```python
from build123d import *

# Parameters (mm, degrees)
SKETCH_R  = 2.5
PAD_DEPTH = 0.8


with BuildPart() as part:
    # Sketch → Pad (new body)
    with BuildSketch(Plane.XY):
        with BuildLine():
            ThreePointArc((-3.20733, 0), (0, -3.20733), (3.20733, 0))
            Line((3.20733, 0), (3.20733, 29.5))
            Line((-3.20733, 29.5), (3.20733, 29.5))
            Line((-3.20733, 0), (-3.20733, 29.5))
        make_face()
        Circle(SKETCH_R, mode=Mode.SUBTRACT)
    extrude(amount=PAD_DEPTH)


solid = part.part
```
Source: CAD feature listing. Evaluate the final solid. Frame: model axes, mm. Give positions to 0.01 mm unless a question says otherwise; leave off trailing zeros. Write each loop counter-clockwise with the first axis right and the second up, starting at its lowest first coordinate (ties: lowest second). Pieces come first, ordered by that corner, then holes.
1. Section query B-B (z = 0.45). Return the cut outline in (x, y), then the cut area to 3 significant figures.
2. Section query A-A (x = 0). Return the cut outline in (y, z), then the cut area to 3 significant figures.
3. Material intervals for line 1 along Y through (x, z) = (0, 0.6); line 2 along Y through (x, z) = (1, 0.3); line 3 along X through (y, z) = (1, 0.7), sorted ascending.
4. Pull-direction query (Y, two-part tool) for faces 1 (the face through (0, 13, 0)), 2 (the face through (-0.54, -2.44, 0.39)), 3 (the face through (-0.071, -3.207, 0.394)); classes: +Y half, -Y half, draft (parallel to the pull), parting line (faces both ways), or undercut.
5. Section query C-C (x = -1.5). Return the cut outline in (y, z).
Output values:
1. outline: (-3.21, 0) arc R3.21 ccw to (3.21, 0) - (3.21, 29.5) - (-3.21, 29.5) - close; hole circle Ø5 at (0, 0)
1. area: 186 mm2
2. outline: (-3.21, 0) - (-2.5, 0) - (-2.5, 0.8) - (-3.21, 0.8) - close; (2.5, 0) - (29.5, 0) - (29.5, 0.8) - (2.5, 0.8) - close
2. area: 22.2 mm2
3. line 1: y = -3.21 to -2.5, 2.5 to 29.5
3. line 2: y = -3.05 to -2.29, 2.29 to 29.5
3. line 3: x = -3.21 to -2.29, 2.29 to 3.21
4. face 1: draft
4. face 2: undercut
4. face 3: -Y half
5. outline: (-2.83, 0) - (-2, 0) - (-2, 0.8) - (-2.83, 0.8) - close; (2, 0) - (29.5, 0) - (29.5, 0.8) - (2, 0.8) - close
